from build123d import *

# Parameters (mm, degrees)
BOSS_EXTRUDE1_DEPTH      = 3.175
SKETCH2_W                = 2.75
SKETCH2_H                = 2.5
SKETCH2_H_2              = 4
SKETCH2_W_2              = 1.125
SKETCH2_H_3              = 7.5
CUT_EXTRUDE1_DEPTH       = 180.884021717
CIRPATTERN1_COUNT        = 4
F_3_0_3_DIAMETER_HOLE1_D = 3
F_1_2_CLEARANCE_HOLE1_D  = 13.89126


with BuildPart() as part:
    # Sketch1 → Boss-Extrude1 (new, symmetric)
    with BuildSketch(Plane(origin=(0, 0, 0), x_dir=(1, 0, 0), z_dir=(0, 1, 0))):
        with BuildLine():
            Line((98.95418457, -7.5), (98.95418457, -150))
            Line((98.95418457, -150), (48.95418457, -150))
            Line((48.95418457, -150), (48.95418457, -86.323047079))
            ThreePointArc((48.95418457, -86.323047079), (-83.800295961, 53.157229431), (98.95418457, -7.5))
        make_face()
        with BuildLine():
            Line((-83.903460262, -7.5), (-15.811388301, -7.5))
            ThreePointArc((-15.811388301, -7.5), (-12.374368671, -12.374368671), (-7.5, -15.811388301))
            Line((-7.5, -15.811388301), (-7.5, -83.903460262))
            ThreePointArc((-7.5, -83.903460262), (-59.565261034, -59.565261034), (-83.903460262, -7.5))
        make_face(mode=Mode.SUBTRACT)
        with BuildLine():
            Line((7.5, -83.903460262), (7.5, -15.811388301))
            ThreePointArc((7.5, -15.811388301), (12.374368671, -12.374368671), (15.811388301, -7.5))
            Line((15.811388301, -7.5), (83.903460262, -7.5))
            ThreePointArc((83.903460262, -7.5), (59.565261034, -59.565261034), (7.5, -83.903460262))
        make_face(mode=Mode.SUBTRACT)
        with BuildLine():
            Line((-83.903460262, 7.5), (-15.811388301, 7.5))
            ThreePointArc((-15.811388301, 7.5), (-12.374368671, 12.374368671), (-7.5, 15.811388301))
            Line((-7.5, 15.811388301), (-7.5, 83.903460262))
            ThreePointArc((-7.5, 83.903460262), (-59.565261034, 59.565261034), (-83.903460262, 7.5))
        make_face(mode=Mode.SUBTRACT)
        with BuildLine():
            Line((7.5, 15.811388301), (7.5, 83.903460262))
            ThreePointArc((7.5, 83.903460262), (59.565261034, 59.565261034), (83.903460262, 7.5))
            Line((83.903460262, 7.5), (15.811388301, 7.5))
            ThreePointArc((15.811388301, 7.5), (12.374368671, 12.374368671), (7.5, 15.811388301))
        make_face(mode=Mode.SUBTRACT)
    extrude(amount=BOSS_EXTRUDE1_DEPTH, both=True)

    # Sketch2 → Cut-Extrude1 (cut, symmetric)
    with BuildSketch(Plane(origin=(0, 0, 0), x_dir=(1, 0, 0), z_dir=(0, 1, 0))):
        with Locations((0, 87.25)):
            Rectangle(SKETCH2_W, SKETCH2_H)
        with Locations((0, 90.5)):
            Rectangle(SKETCH2_W, SKETCH2_H_2)
        with Locations((1.9375, 90.5)):
            Rectangle(SKETCH2_W_2, SKETCH2_H_2)
        with Locations((0, 96.25)):
            Rectangle(SKETCH2_W, SKETCH2_H_3)
        with Locations((-1.9375, 90.5)):
            Rectangle(SKETCH2_W_2, SKETCH2_H_2)
    cut_extrude1 = extrude(amount=CUT_EXTRUDE1_DEPTH, both=True, mode=Mode.SUBTRACT)

    # CirPattern1: Cut-Extrude1 ×4 about axis
    cirpattern1_axis = Axis((0, 0, 0), (0, 1, 0))
    for i in range(1, CIRPATTERN1_COUNT):
        add(cut_extrude1.rotate(cirpattern1_axis, i * 360 / CIRPATTERN1_COUNT), mode=Mode.SUBTRACT)

    # Ø3.0 (3) Diameter Hole1 (through all)
    with Locations(Plane(origin=(0, 3.175, 0), x_dir=(1, 0, 0), z_dir=(0, 1, 0))):
        with Locations((-64.868561892, -64.868561892), (-64.868561892, 64.868561892), (64.868561892, 64.868561892), (64.868561892, -64.868561892)):
            Hole(F_3_0_3_DIAMETER_HOLE1_D / 2)

    # 1/2 Clearance Hole1 (through all)
    with Locations(Plane(origin=(0, 3.175, 0), x_dir=(1, 0, 0), z_dir=(0, 1, 0))):
        with Locations((0, 0)):
            Hole(F_1_2_CLEARANCE_HOLE1_D / 2)


solid = part.part
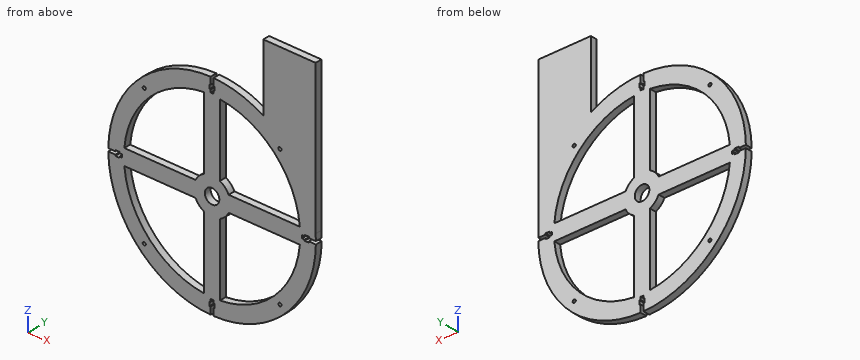
Could you check a few things on this model? Use its own coordinates, in mm. Give positions to 0.01 mm unless a question says otherwise; leave off trailing zeros. Write each loop counter-clockwise with the first axis right and the second up, starting at its lowest first coordinate (ties: lowest second). Pieces come first, ordered by that corner, then holes. Notation, with made-up numbers: (10, 63.25) -> (19, 63.25) arc R19 cw to (19, 69.25) -> close; hole circle Ø3 at (63.25, -34). An arc over 180 degrees is marked (long way). Write each question's results on one line, items separated by ' | '. Start each with the question number.
Q1. Suppose I cut it at C-C, the plane y = -0.75. State how many separate pieces and enclosed holes the cut face has, and give its area (3 significant figures).
Q2. I need wall thicknesses on probe 1 along X at (y, z) = (-1.5, 40.5); probe 2 along X at (y, z) = (2, -52.5); probe 3 along Z at (x, y) = (27, -2.5). Which ranges of each line are inside material? Lowest first, please.
Q3. Suppose I cut it at B-B, the plane z = 56. List the corners of the cut face in (x, y) for me (3 decimals).
Q4. Suppose I cut it at D-D, the plane z = 102. List the corners of the cut face in (x, y) for me (3 decimals), and give its area (4 significant figures).
Q5. Suppose I cut it at A-A, the plane x = -20. List the corners of the cut face in (y, z) for me (3 decimals).
Q6. I'm going to push flat-ended pins straight in: pin 1 Ø1.4 at (x, y) = (0, -1) entering from +Z; pin 2 Ø0.9 at (x, y) = (-2, 1) entering from +Z; pin 3 Ø1.2 at (y, z) = (1.5, 1.5) entering from +X; pin 4 Ø1.2 at (y, z) = (-1, 87) entering from -X. Where does each tip first touch, or does it pass through?
Outcome:
1) separate pieces: 1 | enclosed holes: 9 | area: 17,700 mm2
2) probe 1: -90.6 to -73.86, -7.5 to 7.5, 73.86 to 98.95 | probe 2: -84.21 to -65.88, -7.5 to 7.5, 65.88 to 84.21 | probe 3: -95.49 to -79.79, -7.5 to 7.5, 79.79 to 95.49
3) outline: (-81.928, -3.175) -> (-62.929, -3.175) -> (-62.929, 3.175) -> (-81.928, 3.175) -> close; (-7.5, -3.175) -> (7.5, -3.175) -> (7.5, 3.175) -> (-7.5, 3.175) -> close; (62.929, -3.175) -> (98.954, -3.175) -> (98.954, 3.175) -> (62.929, 3.175) -> close
4) outline: (48.954, -3.175) -> (98.954, -3.175) -> (98.954, 3.175) -> (48.954, 3.175) -> close | area: 317.5 mm2
5) outline: (-3.175, -97.202) -> (3.175, -97.202) -> (3.175, -81.829) -> (-3.175, -81.829) -> close; (-3.175, -7.5) -> (3.175, -7.5) -> (3.175, 7.5) -> (-3.175, 7.5) -> close; (-3.175, 81.829) -> (3.175, 81.829) -> (3.175, 97.202) -> (-3.175, 97.202) -> close
6) pin 1: z = 86 | pin 2: z = 99.23 | pin 3: x = 99.23 | pin 4: x = -48.82
